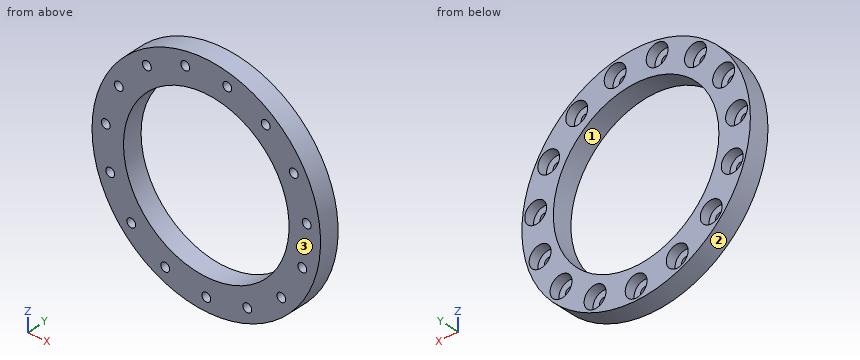
Autodesk Inventor part; units mm, degrees
ref_plane "YZ Plane" through (0, 0, 0) normal (1, 0, 0) x (0, 1, 0)
ref_plane "XZ Plane" through (0, 0, 0) normal (0, 1, 0) x (-1, 0, 0)
ref_plane "XY Plane" through (0, 0, 0) normal (0, 0, 1) x (1, 0, 0)
sketch "Sketch1" plane through (0, 0, 0) normal (0, 1, 0) x (-1, 0, 0)
  circle A0 centre (0, 0) radius 52.9167
  circle A1 centre (0, 0) radius 73.025
  dimension "d0" = 105.8333
  dimension "d1" = 146.05
extrude "Extrusion1" add sketch "Sketch1" against normal blind 12.7
sketch "Sketch2" plane through (0, 0, 0) normal (0, 1, 0) x (1, 0, 0)
  circle A0 centre (0, 64.5584) radius 2.794
  point P0 (0, 0)
  dimension "d5" = 5.588
  dimension "d6" = 64.5584
extrude "Extrusion2" cut sketch "Sketch2" against normal through all
sketch "Sketch3" plane through (0, 0, 0) normal (0, 1, 0) x (1, 0, 0)
  circle A0 centre (0, 64.5584) radius 6.985
  point P0 (0, 0)
  dimension "d9" = 64.5584
  dimension "d10" = 13.97
extrude "Extrusion3" cut sketch "Sketch3" against normal blind 6.35
pattern_circular "Circular Pattern3" count 15 over 360 about axis through (0, 0, 0) along (0, -1, 0) of "Extrusion2", "Extrusion3"
properties part number "wormGearSupport"
The listing builds one solid part. Answer for the finished solid, in the listing's coordinates (mm). Face numbers are marked on the shaded views. Give positions to 0.01 mm unless a question says otherwise; leave off trailing zeros. Loops run counter-clockwise (first coordinate to the right, second up) from the corner with the lowest first, then second, coordinate; pieces in that order, holes last. Notation, with made-up numbers: M 49,-27.75 L 98,-27.75 A15 ccw 98,-3.75 Z; hole C 54.5,48.5 d2. An arc over 180 degrees is marked long. One line per item, written item: value.
Q1. A cutting plane is placed at C-C on z = -29.5. Determine the outline of the cut face in (x, y).
Working result:
outline: M -66.8,-12.7 L -43.93,-12.7 L -43.93,0 L -66.8,0 Z; M 43.93,-12.7 L 66.8,-12.7 L 66.8,0 L 43.93,0 Z
Q2. A cutting plane is placed at A-A on x = 0. Determine the outline of the cut face in (y, z) (3 decimals), then the cut area to 3 significant figures.
Working result:
outline: M -12.7,-73.025 L 0,-73.025 L 0,-71.543 L -6.35,-71.543 L -6.35,-67.352 L -12.7,-67.352 Z; M -12.7,-61.764 L -6.35,-61.764 L -6.35,-57.573 L 0,-57.573 L 0,-52.917 L -12.7,-52.917 Z; M -12.7,52.917 L 0,52.917 L 0,73.025 L -12.7,73.025 Z
area: 387 mm^2
Q3. Find the intervals of material crossed by line 1 (Z direction, x = 0, y = -3.25) (3 decimals); line 2 (Z direction, x = -13.5, y = -4.25); line 3 (Z direction, x = 62, y = -3), in increasing order. Write a range as from..to.
Working result:
line 1: z = -73.025..-71.543, -57.573..-52.917, 52.917..73.025
line 2: z = -71.77..-51.17, 51.17..56.16, 70.13..71.77
line 3: z = -38.58..-26.91, -12.99..0.12, 13.38..28.86, 35.7..38.58
Q4. Determine the mould class of the marked faces 1, 2 and 3 for opening direction Z: +Z half, -Z half, draft (parallel to the pull), parting line (faces both ways), or undercut.
Working result:
face 1: undercut
face 2: parting line
face 3: draft
Q5. Flat-ended cylindrical pins translate along their axes: P1, Ø2, axis at y = -10, z = 51, coming from the +X side; P2, Ø5, axis at x = 20, y = -4.5, coming from the -Z side; P3, Ø4, axis at y = -3, z = 28.5, coming from the +X side. Find the tip coordinate at first contact, or state that the pin passes through.
Working result:
P1: stops at x = 53.22
P2: stops at z = -70.9
P3: stops at x = 68.05
